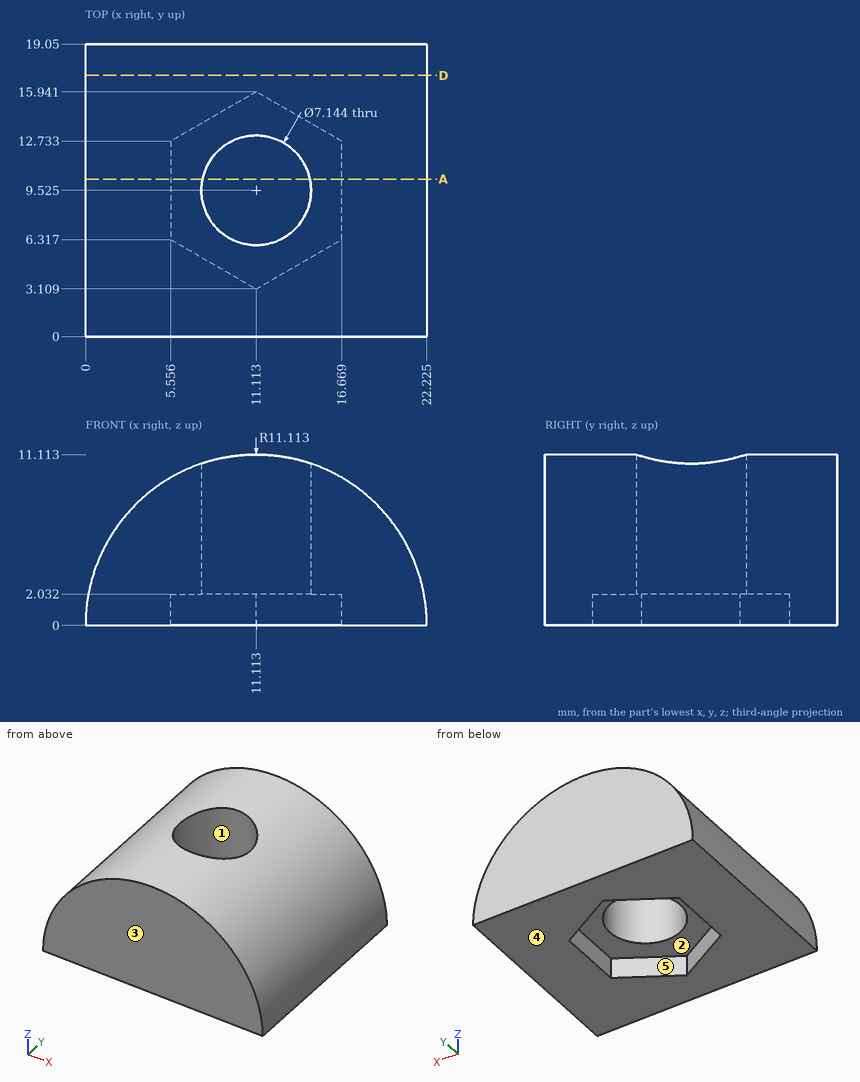
Here's the drawing with two shaded views (mm, measured from the low corner). I have some questions. A direction names the side the tool comes from. Round coordinates to 2 decimals unless told otherwise and drop trailing zeros. Write each loop counter-clockwise with the first axis right and the second up, starting at its lowest first coordinate (ties: lowest second). Pieces come first, ordered by that corner, then holes. Notation, with made-up numbers: M 47.5,48 L 52.5,48 A21 ccw 52.5,83 Z; hole C 27.5,-10.5 d3. An arc over 180 degrees is marked long. Write each question's results on one line, items separated by ' | '. Start each with the question number.
1. Thinking about a two-plate mould opening in Y: for the marked faces 3, 4 and 5, which applies, +Y half, -Y half, draft (parallel to the pull), parting line (faces both ways), or undercut?
2. I'm going to push flat-ended pins straight in: pin 1 Ø3.5 at (x, y) = (10.5, 12) entering from -Z; pin 2 Ø3 at (x, y) = (3, 4) entering from +Z; pin 3 Ø6 at (y, z) = (2, 1.5) entering from +X (1 decimal); pin 4 Ø1 at (x, y) = (17.5, 9.5) entering from +Z (1 decimal). Where does each tip first touch, or does it pass through?
3. Imagine slicing it at A-A on y = 10.25. List the corners of the cut face in (x, z) for me (1 decimal), and give its area (3 significant figures).
4. On a 3-axis mill with a long thin cutter (end or side, diameter ignored), from which of +Z, -Z, +X, -X, +Y, -Y can I reach the whole of each face in a straight line? I mean the marked faces 1 and 2. Say none if no direction works.
5. I need wall thicknesses on L1, parallel to X at y = 7.5, z = 6.25 (1 decimal); L2, parallel to Y at x = 13.5, z = 8; L3, parallel to X at y = 7, z = 4.75 (1 decimal). Which ranges of each line are inside material? Lowest first, please. Write a range as from..to.
6. Imagine slicing it at D-D on y = 17. List the corners of the cut face in (x, z) for me (1 decimal).
Result sheet:
1) face 3: -Y half | face 4: draft | face 5: undercut
2) pin 1: stops at z = 2.03 | pin 2: stops at z = 8.93 | pin 3: stops at x = 22.2 | pin 4: stops at z = 9.4
3) outline: M 0,0 L 5.6,0 L 5.6,2 L 7.6,2 L 7.6,10.5 A11.1 ccw Z; M 14.6,2 L 16.7,2 L 16.7,0 L 22.2,0 A11.1 ccw 14.6,10.5 Z | area: 109 mm^2
4) face 1: +Z, -Z | face 2: -Z
5) L1: x = 1.9..8.2, 14.1..20.3 | L2: y = 0..6.87, 12.18..19.05 | L3: x = 1.1..8.6, 13.6..21.2
6) outline: M 0,0 L 22.2,0 A11.1 ccw Z
